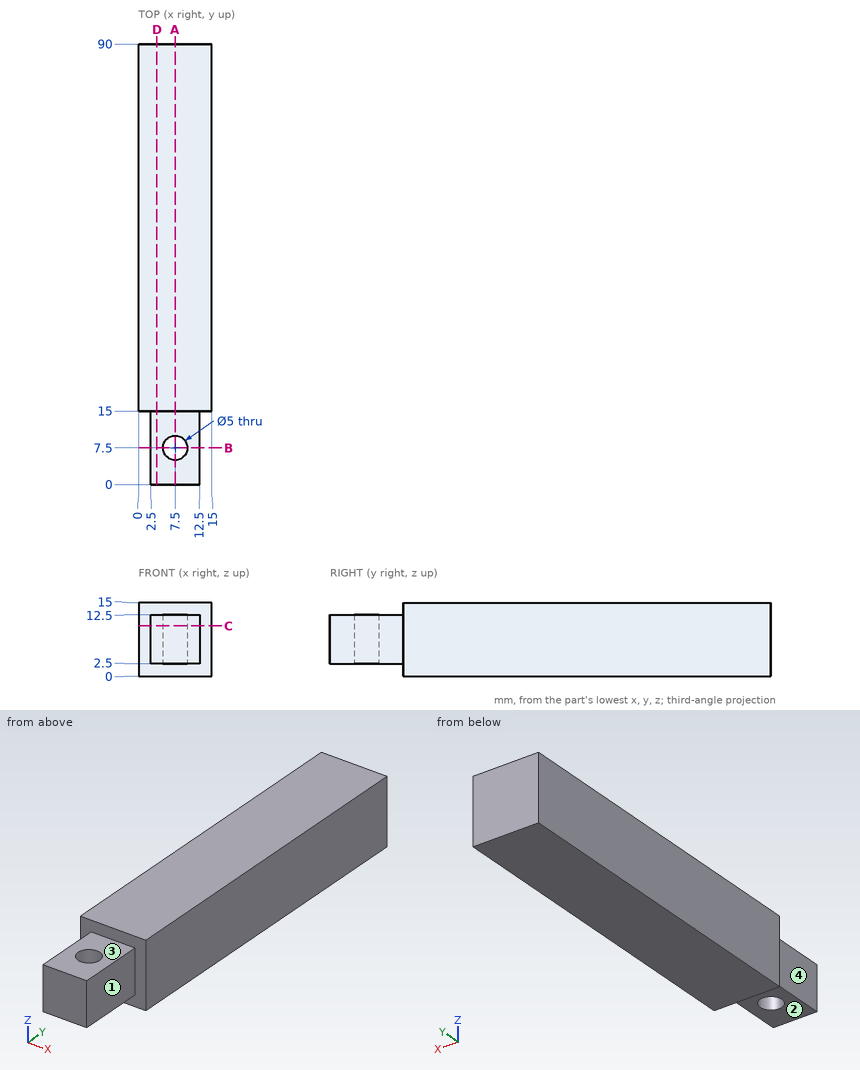
Input: dimensioned drawing with shaded views. Units: mm. Origin: part minimum x, y, z. A direction names the side the tool comes from. Give positions to 0.01 mm unless a question says otherwise; leave off trailing zeros. Order: outer loops, then holes, each group sorted by start corner. A loop starts at its lowest first (then second) coordinate and runs counter-clockwise, first axis right, second up.
(1) Section query D-D (x = 3.75). Return the cut outline in (y, z).
(2) Section query C-C (z = 10.25). Return the cut outline in (x, y), plus the area to 3 significant figures.
(3) Contact query for flat-ended pins moving along their axis: P1, Ø3, axis at y = 7, z = 9, coming from the +X side; P2, Ø6, axis at x = 12, z = 4, coming from the -Y side; P3, Ø3, axis at x = 7.5, y = 7.5, coming from the -Z side; P4, Ø8, axis at x = 8, y = 4.5, coming from the -Z side. Output: stop coordinate, or through.
(4) Material intervals for line 1 along X through (y, z) = (7.5, 8.25); line 2 along Y through (x, z) = (7.5, 6.75); line 3 along Y through (x, z) = (6, 11.25), sorted ascending.
(5) Access query for the marked faces 1, 2, 3 and 4. Directions: +Z, -Z, +X, -X, +Y, -Y. A direction counts if a zero-diameter tool reaches every point of the face in a straight line with its end or side. Return the directions, or none.
(6) Section query A-A (x = 7.5). Return the cut outline in (y, z).
(7) Section query B-B (y = 7.5). Return the cut outline in (x, z).
Outcome:
1. outline: (0, 2.5) - (15, 2.5) - (15, 0) - (90, 0) - (90, 15) - (15, 15) - (15, 12.5) - (0, 12.5) - close
2. outline: (0, 15) - (2.5, 15) - (2.5, 0) - (12.5, 0) - (12.5, 15) - (15, 15) - (15, 90) - (0, 90) - close; hole circle Ø5 at (7.5, 7.5)
2. area: 1,260 mm2
3. P1: stops at x = 12.5
3. P2: stops at y = 0
3. P3: passes through
3. P4: stops at z = 2.5
4. line 1: x = 2.5 to 5, 10 to 12.5
4. line 2: y = 0 to 5, 10 to 90
4. line 3: y = 0 to 5.5, 9.5 to 90
5. face 1: +Z, -Z, +X, -Y
5. face 2: -Z, +X, -X, -Y
5. face 3: +Z, +X, -X, -Y
5. face 4: +Z, -Z, -X, -Y
6. outline: (0, 2.5) - (5, 2.5) - (5, 12.5) - (0, 12.5) - close; (10, 2.5) - (15, 2.5) - (15, 0) - (90, 0) - (90, 15) - (15, 15) - (15, 12.5) - (10, 12.5) - close
7. outline: (2.5, 2.5) - (5, 2.5) - (5, 12.5) - (2.5, 12.5) - close; (10, 2.5) - (12.5, 2.5) - (12.5, 12.5) - (10, 12.5) - close
